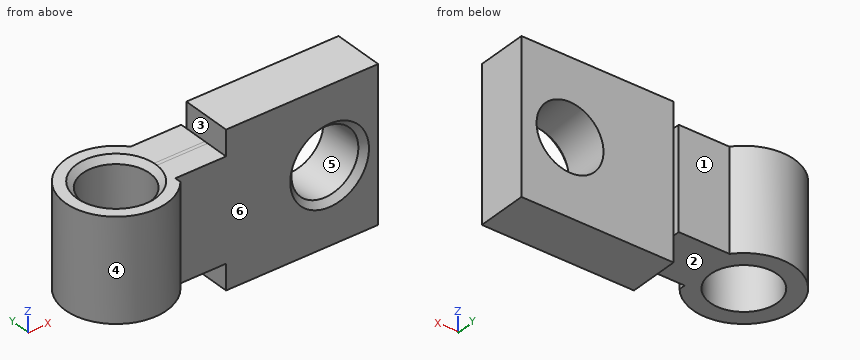
```python
from build123d import *

# Parameters (mm, degrees)
SKETCH_1_R                      = 5
EXTRUDE_1_DEPTH                 = 10
HOLE_WIZARD_G1_16_1_D           = 6.6
HOLE_WIZARD_G1_16_1_DEPTH       = 50
HOLE_WIZARD_G1_16_1_CSINK_D     = 7.773
HOLE_WIZARD_G1_16_1_CSINK_ANGLE = 90
HOLE_WIZARD_G1_16_1_TIP         = 1.982840043
SKETCH_4_W                      = 1.792487356
SKETCH_4_H                      = 9.243284927
CUT_EXTRUDE_1_DEPTH             = 10
EXTRUDE_2_DEPTH                 = 5
SKETCH_6_W                      = 15
SKETCH_6_H                      = 5
EXTRUDE_3_DEPTH                 = 15
HOLE_WIZARD_G1_16_2_D           = 6.6
HOLE_WIZARD_G1_16_2_DEPTH       = 50
HOLE_WIZARD_G1_16_2_CSINK_D     = 7.773
HOLE_WIZARD_G1_16_2_CSINK_ANGLE = 90
HOLE_WIZARD_G1_16_2_TIP         = 1.982840043


with BuildPart() as part:
    # 草图1 → 凸台-拉伸1 (new body)
    with BuildSketch(Plane.XY):
        Circle(SKETCH_1_R)
    extrude(amount=EXTRUDE_1_DEPTH)

    # G1/16 螺纹孔1
    with Locations(Plane.XY.offset(10)):
        with Locations((0, 0)):
            CounterSinkHole(HOLE_WIZARD_G1_16_1_D / 2, HOLE_WIZARD_G1_16_1_CSINK_D / 2, depth=HOLE_WIZARD_G1_16_1_DEPTH, counter_sink_angle=HOLE_WIZARD_G1_16_1_CSINK_ANGLE)
            with Locations((0, 0, -(HOLE_WIZARD_G1_16_1_DEPTH + HOLE_WIZARD_G1_16_1_TIP / 2))):  # 118° drill point
                Cone(0, HOLE_WIZARD_G1_16_1_D / 2, HOLE_WIZARD_G1_16_1_TIP, mode=Mode.SUBTRACT)

    # 草图4 → 切除-拉伸1 (cut)
    with BuildSketch(Plane.XY.offset(10)):
        with Locations((4.778713525, -1.471019051)):
            Rectangle(SKETCH_4_W, SKETCH_4_H)
    extrude(amount=-CUT_EXTRUDE_1_DEPTH, mode=Mode.SUBTRACT)

    # 草图5 → 凸台-拉伸2 (add)
    with BuildSketch(Plane(origin=(3.882469847, 0, 0), x_dir=(0, 0, -1), z_dir=(1, 0, 0))):
        with BuildLine():
            Line((-10, -0.176946718), (-10, -2.5))
            Line((-10, -2.5), (0, -2.5))
            Line((0, -2.5), (0, 3.150623413))
            Line((0, 3.150623413), (-10, 3.150623413))
            Line((-10, 3.150623413), (-10, 0.176946718))
            add(Edge.make_bspline(
                [(-10, 0.176946718), (-9.991943872, 0), (-10, -0.176946718)],
                knots=[-0.045560049, -0.045560049, -0.045560049, 0.045560049, 0.045560049, 0.045560049], degree=2, weights=[1, 1.001038039, 1]))
        make_face()
    extrude(amount=EXTRUDE_2_DEPTH)

    # 草图6 → 凸台-拉伸3 (add)
    with BuildSketch(Plane(origin=(8.882469847, 0, 0), x_dir=(0, 0, -1), z_dir=(1, 0, 0))):
        with Locations((-5, 0)):
            Rectangle(SKETCH_6_W, SKETCH_6_H)
    extrude(amount=EXTRUDE_3_DEPTH)

    # G1/16 螺纹孔2
    with Locations(Plane(origin=(0, -2.5, 0), x_dir=(-1, 0, 0), z_dir=(0, -1, 0))):
        with Locations((-19.093145461, -5)):
            CounterSinkHole(HOLE_WIZARD_G1_16_2_D / 2, HOLE_WIZARD_G1_16_2_CSINK_D / 2, depth=HOLE_WIZARD_G1_16_2_DEPTH, counter_sink_angle=HOLE_WIZARD_G1_16_2_CSINK_ANGLE)
            with Locations((0, 0, -(HOLE_WIZARD_G1_16_2_DEPTH + HOLE_WIZARD_G1_16_2_TIP / 2))):  # 118° drill point
                Cone(0, HOLE_WIZARD_G1_16_2_D / 2, HOLE_WIZARD_G1_16_2_TIP, mode=Mode.SUBTRACT)


solid = part.part
```
The listing builds one solid part. Answer for the finished solid, in the listing's coordinates (mm). Face numbers are marked on the shaded views. A direction names the side the tool comes from. Give positions to 0.01 mm unless a question says otherwise; leave off trailing zeros. Order: outer loops, then holes, each group sorted by start corner. A loop starts at its lowest first (then second) coordinate and runs counter-clockwise, first axis right, second up. Notation, with made-up numbers: (78, 29.25) - (108, 29.25) arc R33 cw to (108, 63.25) - close; hole circle Ø7 at (-14, 78.25). An arc over 180 degrees is marked (long way). Answer in a Markdown table with one row per item. Add a question column.
Q1. The part is cut by section C-C (z = 0.5). Determine the outline of the cut face in (x, y), then the cut area to 3 significant figures.
Q2. The part is cut by section A-A (z = 5). Determine the outline of the cut face in (x, y), then the cut area to 3 significant figures.
Q3. For a pull along X with two mould halves and no side action, classify the marked faces 4, 5 and 6 as released by +X, released by -X, zero draft, split by the parting line, or undercut.
Q4. Which of the six approach directions +Z, -Z, +X, -X, +Y, -Y give full straight-line access (tool end or side, diameter ignored) to the marked faces 1, 2 and 3?
Q5. The part is cut by section B-B (x = 0). Determine the outline of the cut face in (y, z).
Q6. Find the intervals of material crossed by line 1 along X through (y, z) = (0, 6); line 2 along Y through (x, z) = (0, 3.5); line 3 along X through (y, z) = (0, 2.5), in increasing order. Write a range as [from, to].
Q7. Given P1, Ø6, axis at x = 0, y = 0, coming from the -Z side; P2, Ø3, axis at x = 3.5, y = 1, coming from the +Z side; P3, Ø7.5, axis at x = 19.09, z = 5, coming from the -Y side; P4, Ø5, axis at x = -0.5, y = -1, coming from the -Z side, each flat-ended and moving along its own axis, determine where each tip first touches the part or whether it passes through.
Q8. The part is cut by section D-D (y = 0.5). Give the number of separate pieces and of enclosed holes in the cut face, then the cut area to 3 significant figures.
Determined:
| question | item | result |
|---|---|---|
| 1 | outline | (3.88, -3.15) - (3.88, -2.5) - (23.88, -2.5) - (23.88, 2.5) - (8.88, 2.5) - (8.88, 3.15) - (3.88, 3.15) arc R5 ccw (long way) to start; hole circle Ø6.6 at (0, 0) |
| 1 | area | 143 mm² |
| 2 | outline | (3.88, -3.15) - (3.88, -2.5) - (15.21, -2.5) - (15.79, -1.91) - (15.79, 2.5) - (8.88, 2.5) - (8.88, 3.15) - (3.88, 3.15) arc R5 ccw (long way) to start; (22.39, -1.91) - (22.98, -2.5) - (23.88, -2.5) - (23.88, 2.5) - (22.39, 2.5) - close; hole circle Ø6.6 at (0, 0) |
| 2 | area | 109 mm² |
| 3 | face 4 | split by the parting line |
| 3 | face 5 | undercut |
| 3 | face 6 | zero draft |
| 4 | face 1 | +Z, -Z, +X, +Y |
| 4 | face 2 | -Z, -X, +Y, -Y |
| 4 | face 3 | +Z, -X, +Y, -Y |
| 5 | outline | (-5, 0) - (-3.3, 0) - (-3.3, 9.41) - (-3.89, 10) - (-5, 10) - close; (3.3, 0) - (5, 0) - (5, 10) - (3.89, 10) - (3.3, 9.41) - close |
| 6 | line 1 | x = [-5, -3.3], [3.3, 15.95], [22.24, 23.88] |
| 6 | line 2 | y = [-5, -3.3], [3.3, 5] |
| 6 | line 3 | x = [-5, -3.3], [3.3, 16.94], [21.25, 23.88] |
| 7 | P1 | passes through |
| 7 | P2 | stops at z = 10 |
| 7 | P3 | stops at y = -2.37 |
| 7 | P4 | stops at z = 0 |
| 8 | separate pieces | 2 |
| 8 | enclosed holes | 1 |
| 8 | area | 264 mm² |
